from build123d import *

# Parameters (mm, degrees)
BOSS_EXTRUDE1_DEPTH = 3
SKETCH2_R           = 3
CUT_EXTRUDE1_DEPTH  = 5
FILLET1_R           = 5
FILLET3_R           = 1
SKETCH4_R           = 4
SKETCH4_R_2         = 2
BOSS_EXTRUDE2_DEPTH = 2


with BuildPart() as part:
    # Sketch1 → Boss-Extrude1 (new body)
    with BuildSketch(Plane.XY):
        with BuildLine():
            Line((0, -4), (10, -4))
            Line((10, -4), (10, -26))
            Line((10, -26), (15, -26))
            Line((15, -26), (15, 4))
            Line((15, 4), (10, 4))
            Line((10, 4), (0, 4))
            ThreePointArc((0, 4), (-4, 0), (0, -4))
        make_face()
    extrude(amount=BOSS_EXTRUDE1_DEPTH)

    # Sketch2 → Cut-Extrude1 (cut)
    with BuildSketch(Plane(origin=(0, 0, 0), x_dir=(-1, 0, 0), z_dir=(0, 0, -1))):
        Circle(SKETCH2_R)
    extrude(amount=-CUT_EXTRUDE1_DEPTH, mode=Mode.SUBTRACT)

    # Fillet1
    fillet1_edges = [part.edges().sort_by_distance(p)[0] for p in [
        (10, -4, 1.5),
    ]]
    fillet(fillet1_edges, radius=FILLET1_R)

    # Fillet3
    fillet3_edges = [part.edges().sort_by_distance(p)[0] for p in [
        (15, 4, 1.5),
    ]]
    fillet(fillet3_edges, radius=FILLET3_R)

    # Sketch4 → Boss-Extrude2 (add)
    with BuildSketch(Plane(origin=(0, 0, 0), x_dir=(-1, 0, 0), z_dir=(0, 0, -1))):
        Circle(SKETCH4_R)
        Circle(SKETCH4_R_2, mode=Mode.SUBTRACT)
    extrude(amount=BOSS_EXTRUDE2_DEPTH)


solid = part.part
Source: CAD feature listing. Evaluate the final solid. Frame: model axes, mm. A direction names the side the tool comes from. Round coordinates to 2 decimals unless told otherwise and drop trailing zeros. Loops run counter-clockwise (first coordinate to the right, second up) from the corner with the lowest first, then second, coordinate; pieces in that order, holes last.
Q1. First-contact query: P1, Ø0.9, axis at x = 3, z = 2, coming from the -Y side; P2, Ø3, axis at x = 7.5, y = -5.5, coming from the -Z side; P3, Ø0.9, axis at y = -15.5, z = 2, coming from the -X side. Flat tips, straight axial feed; report the tip coordinate or a pass-through.
Q2. Access query for faces 5 (the face through (12, -7, 3)), 6 (the face through (-3.71, 1.49, -0.02)), 7 (the face through (-1, -2, 0)), 8 (the face through (12, -26, 1)), 9 (the face through (2, -4, 1)). Directions: +Z, -Z, +X, -X, +Y, -Y. A direction counts if a zero-diameter tool reaches every point of the face in a straight line with its end or side. Return the directions, or none.
Q3. Ray query, line 1 (Y direction, x = 0, z = -1.15); line 2 (Y direction, x = 0, z = 2.1); line 3 (X direction, y = -2.25, z = 1.9). Return the intervals inside material, ascending.
Q4. Section B-B, the plane z = 1.9. Return loops of the section in (x, y), plus the area to 3 significant figures.
Q5. Section D-D, the plane x = 2.5. Return loops of the section in (y, z).
Q6. Mould query, pull axis Y, two halves, no side actions, for faces 1 (the face through (7, 4, 1)), 2 (the face through (0, -2, -1)), 3 (the face through (10, -17, 1)), 4 (the face through (8, -5, 2)). Classes: pulls with the +Y half, pulls with the -Y half, needs draft (parallel to the pull), parting line crosses it, or undercut.
Q7. Section A-A, the plane y = 0. Return loops of the section in (x, z), plus the area to 3 significant figures.
Q8. Section C-C, the plane x = -0.5. Return loops of the section in (y, z).
Solutions:
1. P1: stops at y = -4
1. P2: stops at z = 0
1. P3: stops at x = 10
2. face 5: +Z, +X, -X, +Y, -Y
2. face 6: -Z
2. face 7: +Z
2. face 8: +Z, -Z, +X, -X, -Y
2. face 9: +Z, -Z, -X, -Y
3. line 1: y = -4 to -2, 2 to 4
3. line 2: y = -4 to -3, 3 to 4
3. line 3: x = -3.31 to -1.98, 1.98 to 15
4. outline: (0, -4) - (5, -4) arc R5 cw to (10, -9) - (10, -26) - (15, -26) - (15, 3) arc R1 ccw to (14, 4) - (0, 4) arc R4 ccw to start; hole circle Ø6 at (0, 0)
4. area: 232 mm2
5. outline: (-4, 0) - (-3.12, 0) - (-3.12, -2) - (3.12, -2) - (3.12, 0) - (4, 0) - (4, 3) - (1.66, 3) - (1.66, 0) - (-1.66, 0) - (-1.66, 3) - (-4, 3) - close
6. face 1: pulls with the +Y half
6. face 2: undercut
6. face 3: needs draft
6. face 4: pulls with the -Y half
7. outline: (-4, -2) - (-2, -2) - (-2, 0) - (-3, 0) - (-3, 3) - (-4, 3) - close; (2, -2) - (4, -2) - (4, 0) - (15, 0) - (15, 3) - (3, 3) - (3, 0) - (2, 0) - close
7. area: 47.0 mm2
8. outline: (-3.97, -2) - (-1.94, -2) - (-1.94, 0) - (-2.96, 0) - (-2.96, 3) - (-3.97, 3) - close; (1.94, -2) - (3.97, -2) - (3.97, 3) - (2.96, 3) - (2.96, 0) - (1.94, 0) - close
